Model file for the job. Use its own axes, mm. A direction names the side the tool comes from. Coordinates: 2 decimals unless noted, no trailing zeros. Write each loop counter-clockwise with the first axis right and the second up, starting at its lowest first coordinate (ties: lowest second). Pieces come first, ordered by that corner, then holes. Notation, with made-up numbers: M 72.25,82 L 110.25,82 A23 cw 110.25,109 Z; hole C 11.25,-34 d10. An arc over 180 degrees is marked long. Put each result on its own line as item: value. Start each with the question number.
Q1. Which spindle directions (+Z, -Z, +X, -X, +Y, -Y) get a long thin tool onto all of the face, cutting with end or side? Do faces 1 (the flat face through (3, -13, -2)), 2 (the flat face through (3, 13, 2)), 3 (the flat face through (3, -2, 13)), 4 (the flat face through (3, -2, -13)). Say none if no direction does.
Q2. Drill centre lines: line 1 along Z through (x, y) = (0.6, 0.25); line 2 along Y through (x, z) = (1.65, 0); line 3 along Z through (x, y) = (2.8, -5). Where is each one in solid material? Low to high.
Q3. Cut at A-A (x = 3.15). Write the cut outline in (y, z), then the cut area to 3 significant figures.
Q4. Drop flat-ended pins along their axis: pin 1 (0.6 mm diameter, centred on x = 1.5, y = 13, fed in from -Z); pin 2 (2 mm diameter, centred on x = 3.5, z = -13, fed in from -Y); pin 3 (1.2 mm diameter, centred on x = 2.5, z = -0.5, fed in from -Y). Give the stop position or say it passes through.
Q5. Pull direction Y, two halves, no side cores. Call faces 5 (the flat face through (3, 0, -12)), 6 (the cylindrical face through (2.9, -9.8, 10)), 7 (the flat face through (0, -8.2, -2.5)): pulls with the +Y half, pulls with the -Y half, needs draft (parallel to the pull), parting line crosses it, or undercut.
Autodesk Inventor part; units mm, degrees
ref_plane "Work Plane1" through (39.9124, 0, 0) normal (0, 1, 0) x (-1, 0, 0)
ref_plane "YZ Plane" through (0, 0, 0) normal (1, 0, 0) x (0, 1, 0)
ref_plane "XZ Plane" through (0, 0, 0) normal (0, 1, 0) x (-1, 0, 0)
sketch "Skizze1" plane through (0, 0, 0) normal (0, 0, 1) x (1, 0, 0)
  line L0 (0, 0) -> (5, 0)
  line L1 (0, 0) -> (0, 14)
  line L2 (0, 14) -> (5, 14)
  line L3 (5, 14) -> (5, 0)
  line L4 (0, 16.8) -> (0, -2.8)
  line L5 (-1, 0) -> (6, 0)
  dimension "d1" = 28
  dimension "d2" = 5
revolve "Körper" add sketch "Skizze1" angle 360 about axis through (0, 0, 0) along (1, 0, 0)
sketch "Skizze2" plane through (0, 0, 0) normal (-1, 0, 0) x (0, 0, 1)
  circle A0 centre (0, 0) radius 14
  point P0 (0, 0)
hole "Gewinde" at (0, 0, 0) direction (1, 0, 0) diameter 15.917 end through all
chamfer "Fase1" distance 2 angle 30 1 edges at (0, -14, 0) measured on face at (0, 11.8312, -1.4366)
sketch "Skizze3" plane through (5, 0, 0) normal (1, 0, 0) x (0, 0, -1)
  circle A0 centre (0, 0) radius 14
  line L0 (-2, 13.8564) -> (-2, 12)
  line L1 (-2, 12) -> (2, 12)
  line L2 (2, 12) -> (2, 13.8564)
  line L3 (0, -19.6) -> (0, 19.6)
  line L4 (-19.6, 0) -> (19.6, 0)
  dimension "d12" = 2
  dimension "d13" = 2
  dimension "d14" = 12
extrude "Nut1" cut sketch "Skizze3" against normal through all contours L2 L1 L3 A0 | L3 L1 L0 A0
pattern_circular "Nuten1" count 4 over 360 about axis through (-10, 0, 0) along (1, 0, 0) of "Nut1"
fillet "Rundung1" radius 0.5 4 edges at (5, 9.8995, 9.8995) (5, 9.8995, -9.8995) (5, -9.8995, -9.8995) (5, -9.8995, 9.8995)
chamfer "Fase2" distance 0.425 angle 45 1 edges at (5, 0, -7.9585) measured on face at (5, -10.6335, 0.3198)
chamfer "Fase3" distance 0.425 angle 45 1 edges at (0, 0, -7.9585) measured on face at (0, 0.8901, -10.5525)
ref_plane "Work Plane1" through (39.9124, 0, 0) normal (0, 1, 0) x (-1, 0, 0)
equation "\"d1\" = SD2"
equation "\"d2\" = KOH"
equation "\"d12\" = 0.5 * SNB"
equation "\"d13\" = 0.5 * SNB"
equation "\"d14\" = 0.5 * SD2 - SNT"
equation "\"d10\" = -0.5 * LADI + 0.5 * SD2"
equation "\"d11\" = FAWI2"
equation "\"d40\" = -0.5 * LADI + 0.5 * SD2"
equation "\"d18\" = RR"
equation "\"d19\" = 0.025 * NND"
equation "\"d41\" = 0.025 * NND"
equation "\"d21\" = 0.025 * NND"
equation "\"d42\" = 0.025 * NND"
equation "\"NND\" = 17"
equation "\"KOH\" = 5"
equation "\"SD2\" = 28"
equation "\"SNB\" = 4"
equation "\"SNT\" = 2"
equation "\"LADI\" = 24"
equation "\"RR\" = 0.5"
equation "\"FAWI2\" = 30deg"
equation "\"GUL\" = 0.61345 * PTC"
equation "\"THREADDIA\" = 17"
equation "\"TOA\" = 30deg"
equation "\"PTC\" = 1"
equation "\"GAL\" = 0.61345 * PTC"
equation "\"GD1\" = THREADDIA - 1.2269 * PTC"
properties part number "DIN 981 - KM 3" material "Stahl, weich"
Computed values:
1. face 1: +X, -X, -Y
1. face 2: +X, -X, +Y
1. face 3: +Z, +X, -X
1. face 4: -Z, +X, -X
2. line 1: -12 to -7.95, 7.95 to 12
2. line 2: -12 to -7.96, 7.96 to 12
2. line 3: -13.08 to -6.19, 6.19 to 13.08
3. outline: M -13.86,-2 A14 ccw -2,-13.86 L -2,-12 L 2,-12 L 2,-13.86 A14 ccw 13.86,-2 L 12,-2 L 12,2 L 13.86,2 A14 ccw 2,13.86 L 2,12 L -2,12 L -2,13.86 A14 ccw -13.86,2 L -12,2 L -12,-2 Z; hole C 0,0 d15.92
3. area: 386 mm2
4. pin 1: z = -5.89
4. pin 2: y = -7.21
4. pin 3: y = -12
5. face 5: undercut
5. face 6: pulls with the -Y half
5. face 7: needs draft
